from build123d import *

# Parameters (mm, degrees)
F0_W     = 1
F0_H     = 22
F0_W_2   = 22
F0_H_2   = 1
F0_W_3   = 44
F0_H_3   = 44
F1_DEPTH = 50
F2_R     = 9
F2_R_2   = 20
F3_DEPTH = 400
F4_R     = 9
F4_R_2   = 20
F5_DEPTH = 400


with BuildPart() as f1:
    # F0 (on Top) → F1 (new body)
    with BuildSketch(Plane.XY):
        with Locations((-45, 34)):
            Rectangle(F0_W, F0_H)
        with Locations((-56.5, 22.5)):
            Rectangle(F0_W_2, F0_H_2)
        with Locations((-22.5, 22.5)):
            Rectangle(F0_W_3, F0_H_2)
        with Locations((-45, 0)):
            Rectangle(F0_W, F0_H_3)
        with Locations((-45, 22.5)):
            Rectangle(F0_W, F0_H_2)
        with Locations((0, 22.5)):
            Rectangle(F0_W, F0_H_2)
        with Locations((0, 34)):
            Rectangle(F0_W, F0_H)
        with Locations((22.5, 22.5)):
            Rectangle(F0_W_3, F0_H_2)
        Rectangle(F0_W, F0_H_3)
        with Locations((45, 22.5)):
            Rectangle(F0_W, F0_H_2)
        with Locations((56.5, 22.5)):
            Rectangle(F0_W_2, F0_H_2)
        with Locations((45, 34)):
            Rectangle(F0_W, F0_H)
        with Locations((45, 0)):
            Rectangle(F0_W, F0_H_3)
        with Locations((56.5, -22.5)):
            Rectangle(F0_W_2, F0_H_2)
        with Locations((45, -34)):
            Rectangle(F0_W, F0_H)
        with Locations((45, -22.5)):
            Rectangle(F0_W, F0_H_2)
        with Locations((22.5, -22.5)):
            Rectangle(F0_W_3, F0_H_2)
        with Locations((0, -22.5)):
            Rectangle(F0_W, F0_H_2)
        with Locations((0, -34)):
            Rectangle(F0_W, F0_H)
        with Locations((-22.5, -22.5)):
            Rectangle(F0_W_3, F0_H_2)
        with Locations((-56.5, -22.5)):
            Rectangle(F0_W_2, F0_H_2)
        with Locations((-45, -34)):
            Rectangle(F0_W, F0_H)
        with Locations((-45, -22.5)):
            Rectangle(F0_W, F0_H_2)
    extrude(amount=F1_DEPTH)

    # F2 (on face) → F3 (cut)
    with BuildSketch(Plane.XZ.offset(23)):
        with Locations((-56.5, 34)):
            Circle(F2_R)
        with Locations((-67.5, 0)):
            Circle(F2_R_2)
        with BuildLine():
            Line((-42.5, 0), (-2.5, 0))
            ThreePointArc((-2.5, 0), (-22.5, 20), (-42.5, 0))
        make_face()
        with Locations((-32.5, 34)):
            Circle(F2_R)
        with Locations((-12.5, 34)):
            Circle(F2_R)
        with Locations((22.5, 0)):
            Circle(F2_R_2)
        with Locations((12.5, 34)):
            Circle(F2_R)
        with Locations((32.5, 34)):
            Circle(F2_R)
        with Locations((56.5, 34)):
            Circle(F2_R)
        with Locations((67.5, 0)):
            Circle(F2_R_2)
    extrude(amount=-F3_DEPTH, mode=Mode.SUBTRACT)

    # F4 (on face) → F5 (cut)
    with BuildSketch(Plane.YZ.offset(45.5)):
        with Locations((-34, 34)):
            Circle(F4_R)
        with Locations((-10, 34)):
            Circle(F4_R)
        with Locations((10, 34)):
            Circle(F4_R)
        with Locations((34, 34)):
            Circle(F4_R)
        with Locations((45, 0)):
            Circle(F4_R_2)
        with BuildLine():
            Line((-20, 0), (20, 0))
            ThreePointArc((20, 0), (0, 20), (-20, 0))
        make_face()
        with Locations((-45, 0)):
            Circle(F4_R_2)
    extrude(amount=-F5_DEPTH, mode=Mode.SUBTRACT)


solid = f1.part
Verification items for the finished model (mm, model axes). A direction names the side the tool comes from. Coordinates: 2 decimals unless noted, no trailing zeros. Write each loop counter-clockwise with the first axis right and the second up, starting at its lowest first coordinate (ties: lowest second). Pieces come first, ordered by that corner, then holes. Notation, with made-up numbers: (65.25, 59.25) - (88.25, 59.25) arc R18 ccw to (88.25, 78.25) - close; hole circle Ø3 at (35.25, -35.5). An arc over 180 degrees is marked (long way). Answer as a JSON object with one key per item and string values.
(1) Gauge pin test, flat ends, axial feed: pin 1 Ø6 at (y, z) = (-13, 35.5) entering from -X; pin 2 Ø20.5 at (y, z) = (-10, 34) entering from -X; pin 3 Ø8 at (y, z) = (3.5, 17) entering from +X; pin 4 Ø6 at (x, z) = (46.5, 12.5) entering from -Y. Record the tip position at first contact, or that the pin passes through.
Report:
{"pin 1": "through", "pin 2": "x = -45.5", "pin 3": "x = 45.5", "pin 4": "y = -32.15"}
(2) Tool access check on faces 1 (the flat face through (-45.5, 31, 25)), 2 (the flat face through (-0.5, 31, 25)), 3 (the flat face through (44.5, -31, 25)), 4 (the cylindrical face through (-51.66, -22.51, 41.59)), 5 (the flat face through (54, -22, 25)). Record the directions out of +Z, -Z, +X, -X, +Y, -Y that give a thin tool (end or side, any length) a straight path to the whole face; none if there is none.
Report:
{"face 1": "+Z, -Z, -X, +Y", "face 2": "+Z, -Z, +Y", "face 3": "+Z, -Z, -Y", "face 4": "+Y, -Y", "face 5": "+Z, -Z, +X"}
(3) Cross-section at D-D on y = 3.5. Record the cut outline in (x, z).
Report:
{"outline": "(-45.5, 19.69) - (-44.5, 19.69) - (-44.5, 27.78) - (-45.5, 27.78) - close; (-45.5, 40.22) - (-44.5, 40.22) - (-44.5, 50) - (-45.5, 50) - close; (-0.5, 19.69) - (0.5, 19.69) - (0.5, 27.78) - (-0.5, 27.78) - close; (-0.5, 40.22) - (0.5, 40.22) - (0.5, 50) - (-0.5, 50) - close; (44.5, 19.69) - (45.5, 19.69) - (45.5, 27.78) - (44.5, 27.78) - close; (44.5, 40.22) - (45.5, 40.22) - (45.5, 50) - (44.5, 50) - close"}
(4) Mould release check, pull along Z, two halves, no side actions. Record for faces 6 (the cylindrical face through (0.01, 14.84, 41.59)), 7 (the flat face through (-23, -22, 30)), 8 (the cylindrical face through (-22.06, -22.507, 19.995)): pulls with the +Z half, pulls with the -Z half, needs draft (parallel to the pull), parting line crosses it, or undercut.
Report:
{"face 6": "undercut", "face 7": "needs draft", "face 8": "pulls with the -Z half"}
(5) Thickness scan on line 1 along X through (y, z) = (-40, 46); line 2 along Y through (x, z) = (51, 18); line 3 along Z through (x, y) = (-32.5, 22.3). Record the ranges inside material, lowest first.
Report:
{"line 1": "-45.5 to -44.5, -0.5 to 0.5, 44.5 to 45.5", "line 2": "-23 to -22, 22 to 23", "line 3": "17.32 to 25, 43 to 50"}
(6) Cross-section at B-B on y = 13. Record the cut outline in (x, z).
Report:
{"outline": "(-45.5, 15.2) - (-44.5, 15.2) - (-44.5, 25.51) - (-45.5, 25.51) - close; (-45.5, 42.49) - (-44.5, 42.49) - (-44.5, 50) - (-45.5, 50) - close; (-0.5, 15.2) - (0.5, 15.2) - (0.5, 25.51) - (-0.5, 25.51) - close; (-0.5, 42.49) - (0.5, 42.49) - (0.5, 50) - (-0.5, 50) - close; (44.5, 15.2) - (45.5, 15.2) - (45.5, 25.51) - (44.5, 25.51) - close; (44.5, 42.49) - (45.5, 42.49) - (45.5, 50) - (44.5, 50) - close"}
(7) Cross-section at A-A on x = 56.5. Record the cut outline in (y, z), plus the area to 3 significant figures.
Report:
{"outline": "(-23, 16.7) - (-22, 16.7) - (-22, 25) - (-23, 25) - close; (-23, 43) - (-22, 43) - (-22, 50) - (-23, 50) - close; (22, 16.7) - (23, 16.7) - (23, 25) - (22, 25) - close; (22, 43) - (23, 43) - (23, 50) - (22, 50) - close", "area": "30.6 mm^2"}
(8) Cross-section at C-C on z = 34. Give the number of separate pieces and of enclosed holes in the cut face, plus the area to 3 significant figures.
Report:
{"separate pieces": "23", "enclosed holes": "0", "area": "102 mm^2"}
